Design review of the part shown in the three views and the two pictorial views. Dimensions are in mm from the part's minimum x, y and z. A direction names the side the tool comes from. Coordinates: 2 decimals unless noted, no trailing zeros. Loops run counter-clockwise (first coordinate to the right, second up) from the corner with the lowest first, then second, coordinate; pieces in that order, holes last. Notation, with made-up numbers: (83.25, 44.5) -> (132.25, 44.5) arc R35 ccw to (132.25, 79.5) -> close; hole circle Ø6 at (47.25, -3.5). An arc over 180 degrees is marked (long way). Answer in a Markdown table with one row per item.
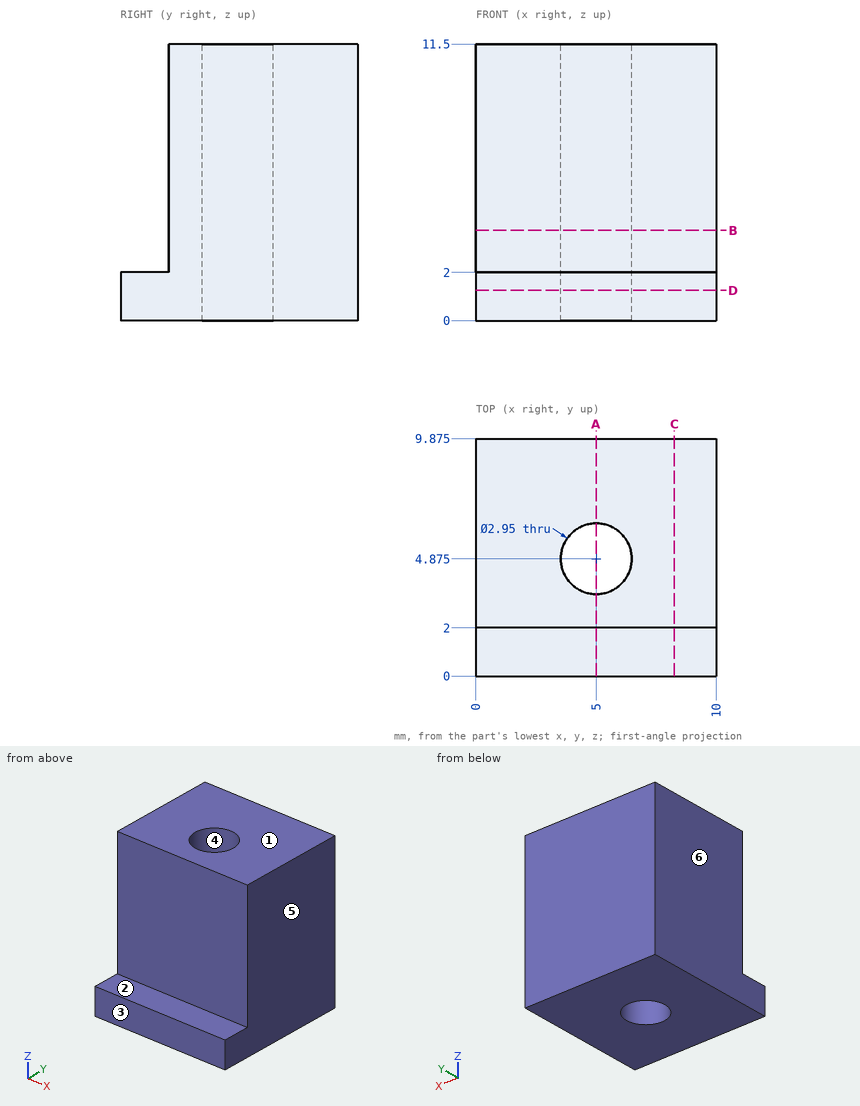
(1) Tool access review of the marked faces 1 and 2: name each direction out of +Z, -Z, +X, -X, +Y, -Y from which nothing blocks a thin tool from reaching the whole face with its end or side.
Evaluation:
| item | result |
|---|---|
| face 1 | +Z, +X, -X, +Y, -Y |
| face 2 | +Z, +X, -X, -Y |
(2) Draft analysis for pull direction X (two halves, no side actions). For the marked faces 3, 4, 5 and 6, state which applies: pulls with the +X half, pulls with the -X half, needs draft (parallel to the pull), parting line crosses it, or undercut.
Evaluation:
| item | result |
|---|---|
| face 3 | needs draft |
| face 4 | undercut |
| face 5 | pulls with the +X half |
| face 6 | pulls with the -X half |
(3) Take a section at A-A on x = 5. Give the boundary of the cut face in (y, z) (3 decimals).
Evaluation:
| item | result |
|---|---|
| outline | (0, 0) -> (3.4, 0) -> (3.4, 11.5) -> (2, 11.5) -> (2, 2) -> (0, 2) -> close; (6.35, 0) -> (9.875, 0) -> (9.875, 11.5) -> (6.35, 11.5) -> close |
(4) For pin 1 (5 mm diameter, centred on x = 3, z = 5, fed in from -Y); pin 2 (1.6 mm diameter, centred on x = 4.5, y = 1, fed in from +Z), all flat-tipped, find the tip position at first contact; note any pin that passes through.
Evaluation:
| item | result |
|---|---|
| pin 1 | stops at y = 2 |
| pin 2 | stops at z = 2 |
(5) Take a section at B-B on z = 3.75. Give the boundary of the cut face in (x, y) (3 decimals).
Evaluation:
| item | result |
|---|---|
| outline | (0, 2) -> (10, 2) -> (10, 9.875) -> (0, 9.875) -> close; hole circle Ø2.95 at (5, 4.875) |
(6) Take a section at D-D on z = 1.25. Give the boundary of the cut face in (x, y) (3 decimals).
Evaluation:
| item | result |
|---|---|
| outline | (0, 0) -> (10, 0) -> (10, 9.875) -> (0, 9.875) -> close; hole circle Ø2.95 at (5, 4.875) |
(7) Take a section at C-C on x = 8.25. Give the boundary of the cut face in (y, z) (3 decimals), and give its area (3 significant figures).
Evaluation:
| item | result |
|---|---|
| outline | (0, 0) -> (9.875, 0) -> (9.875, 11.5) -> (2, 11.5) -> (2, 2) -> (0, 2) -> close |
| area | 94.6 mm² |
(8) To check wall thickness, follow probe 1 along Y at (x, z) = (5, 6) (3 decimals); probe 2 along Y at (x, z) = (7.25, 9) (3 decimals); probe 3 along Z at (x, y) = (5, 1.75). State the ranges of each line that lie inside material, in increasing order.
Evaluation:
| item | result |
|---|---|
| probe 1 | y = 2 to 3.4, 6.35 to 9.875 |
| probe 2 | y = 2 to 9.875 |
| probe 3 | z = 0 to 2 |
